The listing builds one solid part. Answer for the finished solid, in the listing's coordinates (mm). A direction names the side the tool comes from. Round coordinates to 2 decimals unless told otherwise and drop trailing zeros. Write each loop counter-clockwise with the first axis right and the second up, starting at its lowest first coordinate (ties: lowest second). Pieces come first, ordered by that corner, then holes. Notation, with made-up numbers: (38.5, 69) - (93.5, 69) arc R25 ccw to (93.5, 102) - close; hole circle Ø5 at (-33.75, 21). An arc over 180 degrees is marked (long way). Use a Markdown table: item, result. Add a question column.
1) Determine the mould class of faces 1 (the flat face through (4, 0, 6.8)), 2 (the flat face through (9.22, 0, 3)), 3 (the flat face through (3.465, 0, 3)) for opening direction X: +X half, -X half, draft (parallel to the pull), parting line (faces both ways), or undercut.
2) A tool of negligible diameter and unlimited length cuts with its end or side. For faces 4 (the flat face through (4, -1.2, 3)), 5 (the flat face through (5, -0.7, 3)), from which of +Z, -Z, +X, -X, +Y, -Y can it reach the whole face along a straight path? Write none if from no direction.
3) Find the intervals of material crossed by probe 1 along X at (y, z) = (-0.3, 0.75) (3 decimals); probe 2 along Y at (x, z) = (2.5, 0.75); probe 3 along X at (y, z) = (-0.3, 6.75), in increasing order. Write a range as from..to.
4) A cutting plane is placed at C-C (y = -0.1). State how many separate pieces and enclosed holes the cut face has, then the cut area to 3 significant figures.
5) A cutting plane is placed at B-B (z = 5). Give the vertices of the cut face in (x, y) (3 decimals).
6) A cutting plane is placed at A-A (x = 0.25). Give the vertices of the cut face in (y, z), then the cut area to 3 significant figures.
```python
from build123d import *

# Parameters (mm, degrees)
SKETCH007_W      = 1
SKETCH007_H      = 1
EXTRUDE007_DEPTH = 9
SKETCH008_W      = 4
SKETCH008_H      = 1.4
EXTRUDE008_DEPTH = 0.5
SKETCH006_W      = 1.85
SKETCH006_H      = 1.4
EXTRUDE006_DEPTH = 6.3
SKETCH005_W      = 3.2
SKETCH005_H      = 2.4
EXTRUDE005_DEPTH = 6.8
CHAMFER001_SIZE  = 0.4
ARRAY003_X_COUNT = 4
ARRAY003_X_PITCH = 2.54


with BuildPart() as extrude007:
    # Sketch007 → Extrude007 (new body)
    with BuildSketch(Plane.XY):
        Rectangle(SKETCH007_W, SKETCH007_H)
    extrude(amount=EXTRUDE007_DEPTH)


with BuildPart() as extrude008:
    # Sketch008 → Extrude008 (new body)
    with BuildSketch(Plane.XY):
        Rectangle(SKETCH008_W, SKETCH008_H)
    extrude(amount=EXTRUDE008_DEPTH)


with BuildPart() as fusion002:
    # Sketch006 → Extrude006 (new body)
    with BuildSketch(Plane.XY):
        Rectangle(SKETCH006_W, SKETCH006_H)
    extrude(amount=EXTRUDE006_DEPTH)

    # Fusion002: union Extrude007, Extrude008
    add(extrude007.part)
    add(extrude008.part)


with BuildPart() as body001:
    # Sketch005 → Extrude005 (new body)
    with BuildSketch(Plane.XY):
        Rectangle(SKETCH005_W, SKETCH005_H)
    extrude(amount=EXTRUDE005_DEPTH)

    # Cut002: cut Fusion002
    add(fusion002.part, mode=Mode.SUBTRACT)

    # Chamfer001
    chamfer001_edges = [body001.edges().sort_by_distance(p)[0] for p in [
        (0.5, 0, 6.8),
        (0, 0.5, 6.8),
        (-0.5, 0, 6.8),
        (0, -0.5, 6.8),
    ]]
    chamfer(chamfer001_edges, length=CHAMFER001_SIZE)

    # Array003 X: body001 ×4


with BuildPart() as body001_1:
    add(body001.part)
    with Locations(*[(i * ARRAY003_X_PITCH, 0, 0) for i in range(1, ARRAY003_X_COUNT)]):
        add(body001.part)


solid = body001_1.part
```
Entries:
| question | item | result |
|---|---|---|
| 1 | face 1 | draft |
| 1 | face 2 | +X half |
| 1 | face 3 | undercut |
| 2 | face 4 | +Z, -Z, +X, -X, -Y |
| 2 | face 5 | -Z |
| 3 | probe 1 | x = -1.6..-0.925, 0.925..1.615, 3.465..4.155, 6.005..6.695, 8.545..9.22 |
| 3 | probe 2 | y = -1.2..-0.7, 0.7..1.2 |
| 3 | probe 3 | x = -1.6..-0.85, 0.85..1.69, 3.39..4.23, 5.93..6.77, 8.47..9.22 |
| 4 | separate pieces | 5 |
| 4 | enclosed holes | 0 |
| 4 | area | 22.6 mm² |
| 5 | outline | (-1.6, -1.2) - (9.22, -1.2) - (9.22, 1.2) - (-1.6, 1.2) - close; hole (-0.925, -0.7) - (0.925, -0.7) - (0.925, 0.7) - (-0.925, 0.7) - close; hole (1.615, -0.7) - (3.465, -0.7) - (3.465, 0.7) - (1.615, 0.7) - close; hole (4.155, -0.7) - (6.005, -0.7) - (6.005, 0.7) - (4.155, 0.7) - close; hole (6.695, -0.7) - (8.545, -0.7) - (8.545, 0.7) - (6.695, 0.7) - close |
| 6 | outline | (-1.2, 0) - (-0.7, 0) - (-0.7, 6.3) - (-0.5, 6.3) - (-0.5, 6.4) - (-0.9, 6.8) - (-1.2, 6.8) - close; (0.5, 6.3) - (0.7, 6.3) - (0.7, 0) - (1.2, 0) - (1.2, 6.8) - (0.9, 6.8) - (0.5, 6.4) - close |
| 6 | area | 6.84 mm² |
